Read the model definition and answer for the solid it produces. Units are mm, in the model's axes. Face numbers are marked on the shaded views. Coordinates: 2 decimals unless noted, no trailing zeros. Order: outer loops, then holes, each group sorted by start corner. A loop starts at its lowest first (then second) coordinate and runs counter-clockwise, first axis right, second up.
from build123d import *

# Parameters (mm, degrees)
SKETCH_1_W           = 52
SKETCH_1_H           = 95
EXTRUDE_1_DEPTH      = 180
SKETCH_2_W           = 23
SKETCH_2_H           = 90
CUT_EXTRUDE_1_DEPTH  = 140
SKETCH_3_W           = 9.5
SKETCH_3_H           = 2.2
CUT_EXTRUDE_2_DEPTH  = 140
CHAMFER_1_SIZE       = 2
CUT_EXTRUDE_3_DEPTH  = 140
SKETCH_5_W           = 140
SKETCH_5_H           = 15
CUT_EXTRUDE_4_DEPTH  = 140
SKETCH_6_W           = 140
SKETCH_6_H           = 15
CUT_EXTRUDE_7_DEPTH  = 140
CUT_EXTRUDE_8_DEPTH  = 140
SKETCH_8_W           = 24.808453611
SKETCH_8_H           = 15
CUT_EXTRUDE_9_DEPTH  = 140
SKETCH_9_W           = 10
SKETCH_9_H           = 14.176065277
SKETCH_9_H_2         = 15.630765607
CUT_EXTRUDE_10_DEPTH = 140
SKETCH_10_W          = 52
SKETCH_10_H          = 0.823934723
CUT_EXTRUDE_11_DEPTH = 10
SKETCH_12_R          = 3.01
EXTRUDE_2_DEPTH      = 20
CHAMFER_3_SIZE       = 0.5
SKETCH_13_R          = 3.01
EXTRUDE_4_DEPTH      = 20
CHAMFER_4_SIZE       = 0.5
EXTRUDE_START        = 20
SKETCH_15_R          = 3.01
EXTRUDE_5_DEPTH      = 20
CHAMFER_5_SIZE       = 0.5


with BuildPart() as part:
    # 草图1 → 凸台-拉伸1 (new body)
    with BuildSketch(Plane.XY):
        with Locations((0, 47.5)):
            Rectangle(SKETCH_1_W, SKETCH_1_H)
    extrude(amount=EXTRUDE_1_DEPTH)

    # 草图2 → 切除-拉伸1 (cut)
    with BuildSketch(Plane(origin=(0, 0, 0), x_dir=(-1, 0, 0), z_dir=(0, 0, -1))):
        with Locations((0, 50)):
            Rectangle(SKETCH_2_W, SKETCH_2_H)
    extrude(amount=-CUT_EXTRUDE_1_DEPTH, mode=Mode.SUBTRACT)

    # 草图3 → 切除-拉伸2 (cut)
    with BuildSketch(Plane(origin=(0, 0, 0), x_dir=(-1, 0, 0), z_dir=(0, 0, -1))):
        with Locations((-16.25, 6.1)):
            Rectangle(SKETCH_3_W, SKETCH_3_H)
        with Locations((16.25, 6.1)):
            Rectangle(SKETCH_3_W, SKETCH_3_H)
    extrude(amount=-CUT_EXTRUDE_2_DEPTH, mode=Mode.SUBTRACT)

    # 倒角1
    chamfer_1_edges = [part.edges().sort_by_distance(p)[0] for p in [
        (11.5, 51.1, 140),
        (0, 95, 140),
        (11.5, 95, 70),
        (-11.5, 95, 70),
        (11.5, 51.1, 0),
        (-11.5, 51.1, 140),
        (-11.5, 51.1, 0),
        (11.5, 7.2, 70),
        (16.25, 7.2, 140),
        (-16.25, 7.2, 140),
        (-11.5, 7.2, 70),
    ]]
    chamfer(chamfer_1_edges, length=CHAMFER_1_SIZE)

    # 草图4 → 切除-拉伸3 (cut)
    with BuildSketch(Plane(origin=(0, 0, 0), x_dir=(-1, 0, 0), z_dir=(0, 0, -1))):
        Polygon((-0.565514489, 0), (0, 0), (12.126296858, 0), (12.126296858, 5), (-11.873703142, 5), (-11.873703142, 0), align=None)
    extrude(amount=-CUT_EXTRUDE_3_DEPTH, mode=Mode.SUBTRACT)

    # 草图5 → 切除-拉伸4 (cut)
    with BuildSketch(Plane(origin=(26, 0, 0), x_dir=(0, 0, -1), z_dir=(1, 0, 0))):
        with Locations((-70, 87.5)):
            Rectangle(SKETCH_5_W, SKETCH_5_H)
    extrude(amount=-CUT_EXTRUDE_4_DEPTH, mode=Mode.SUBTRACT)

    # 草图6 → 切除-拉伸7 (cut)
    with BuildSketch(Plane(origin=(26, 0, 0), x_dir=(0, 0, -1), z_dir=(1, 0, 0))):
        with Locations((-70, 16.784197303)):
            Rectangle(SKETCH_6_W, SKETCH_6_H)
    extrude(amount=-CUT_EXTRUDE_7_DEPTH, mode=Mode.SUBTRACT)

    # 草图7 → 切除-拉伸8 (cut)
    with BuildSketch(Plane(origin=(0, 95, 0), x_dir=(1, 0, 0), z_dir=(0, 1, 0))):
        Polygon((0, -140), (21.6540992, -140), (21.6540992, -164.808453611), (-20.3459008, -164.808453611), (-20.926391083, -164.808453611), (-20.926391083, -140), align=None)
    extrude(amount=-CUT_EXTRUDE_8_DEPTH, mode=Mode.SUBTRACT)

    # 草图8 → 切除-拉伸9 (cut)
    with BuildSketch(Plane(origin=(26, 0, 0), x_dir=(0, 0, -1), z_dir=(1, 0, 0))):
        with Locations((-152.404226806, 87.5)):
            Rectangle(SKETCH_8_W, SKETCH_8_H)
        with Locations((-152.404226806, 16.784197303)):
            Rectangle(SKETCH_8_W, SKETCH_8_H)
    extrude(amount=-CUT_EXTRUDE_9_DEPTH, mode=Mode.SUBTRACT)

    # 草图9 → 切除-拉伸10 (cut)
    with BuildSketch(Plane(origin=(26, 0, 0), x_dir=(0, 0, -1), z_dir=(1, 0, 0))):
        with Locations((-169.808453611, 87.911967362)):
            Rectangle(SKETCH_9_W, SKETCH_9_H)
        with Locations((-169.808453611, 17.099580106)):
            Rectangle(SKETCH_9_W, SKETCH_9_H_2)
    extrude(amount=-CUT_EXTRUDE_10_DEPTH, mode=Mode.SUBTRACT)

    # 草图10 → 切除-拉伸11 (cut)
    with BuildSketch(Plane(origin=(0, 0, 164.808453611), x_dir=(-1, 0, 0), z_dir=(0, 0, -1))):
        with Locations((0, 80.411967362)):
            Rectangle(SKETCH_10_W, SKETCH_10_H)
    extrude(amount=-CUT_EXTRUDE_11_DEPTH, mode=Mode.SUBTRACT)

    # 草图12 → 凸台-拉伸2 (add)
    with BuildSketch(Plane.XY.offset(180)):
        with Locations(Location((0, 3.01, 0), (0, 0, 270))):
            Circle(SKETCH_12_R)
    extrude(amount=EXTRUDE_2_DEPTH)

    # 倒角3
    chamfer_3_edges = [part.edges().sort_by_distance(p)[0] for p in [
        (0, 6.02, 200),
    ]]
    chamfer(chamfer_3_edges, length=CHAMFER_3_SIZE)

    # 草图13 → 凸台-拉伸4 (add)
    with BuildSketch(Plane(origin=(26, 0, 0), x_dir=(0, 0, -1), z_dir=(1, 0, 0))):
        with Locations(Location((-25, 3.01, 0), (0, 0, 270))):
            Circle(SKETCH_13_R)
    extrude(amount=EXTRUDE_4_DEPTH)

    # 倒角4
    # the kernel refuses this chamfer: 0.5 mm, written as the material it adds along each edge
    with BuildSketch(Plane(origin=(26, 3.01, 25), x_dir=(0, -1, 0), z_dir=(0, 0, 1))) as chamfer_4_piece_1_section:
        Polygon((3.01 + CHAMFER_4_SIZE, 0), (3.01, CHAMFER_4_SIZE), (3.01, 0), align=None)
    chamfer_4_piece_1 = revolve(axis=Axis((26, 3.01, 25), (1, 0, 0)), mode=Mode.PRIVATE)
    chamfer_4_piece_1 = split(chamfer_4_piece_1, bisect_by=Plane(origin=(26.240420809, 0, 25), z_dir=(0, 1, 0)), keep=Keep.TOP, mode=Mode.PRIVATE)
    add(chamfer_4_piece_1)
    # the kernel refuses this chamfer: 0.5 mm, written as the material it takes off along each edge
    with BuildSketch(Plane(origin=(46, 3.01, 25), x_dir=(0, -1, 0), z_dir=(0, 0, 1))) as chamfer_4_2_piece_1:
        Polygon((3.01, -CHAMFER_4_SIZE), (3.01 - CHAMFER_4_SIZE, 0), (3.01, 0), align=None)
    revolve(axis=Axis((46, 3.01, 25), (1, 0, 0)), mode=Mode.SUBTRACT)

    # 草图15 → 凸台-拉伸5 (add)
    with BuildSketch(Plane.ZY.offset(26).offset(EXTRUDE_START)):
        with Locations(Location((25, 3.01, 0), (0, 0, 270))):
            Circle(SKETCH_15_R)
    extrude(amount=-EXTRUDE_5_DEPTH)

    # 倒角5
    # the kernel refuses this chamfer: 0.5 mm, written as the material it adds along each edge
    with BuildSketch(Plane(origin=(-26, 3.01, 25), x_dir=(0, -1, 0), z_dir=(0, 0, -1))) as chamfer_5_piece_1_section:
        Polygon((3.01 + CHAMFER_5_SIZE, 0), (3.01, CHAMFER_5_SIZE), (3.01, 0), align=None)
    chamfer_5_piece_1 = revolve(axis=Axis((-26, 3.01, 25), (-1, 0, 0)), mode=Mode.PRIVATE)
    chamfer_5_piece_1 = split(chamfer_5_piece_1, bisect_by=Plane(origin=(-26.240420809, 0, 25), z_dir=(0, 1, 0)), keep=Keep.TOP, mode=Mode.PRIVATE)
    add(chamfer_5_piece_1)
    # the kernel refuses this chamfer: 0.5 mm, written as the material it takes off along each edge
    with BuildSketch(Plane(origin=(-46, 3.01, 25), x_dir=(0, -1, 0), z_dir=(0, 0, -1))) as chamfer_5_2_piece_1:
        Polygon((3.01, -CHAMFER_5_SIZE), (3.01 - CHAMFER_5_SIZE, 0), (3.01, 0), align=None)
    revolve(axis=Axis((-46, 3.01, 25), (-1, 0, 0)), mode=Mode.SUBTRACT)


solid = part.part
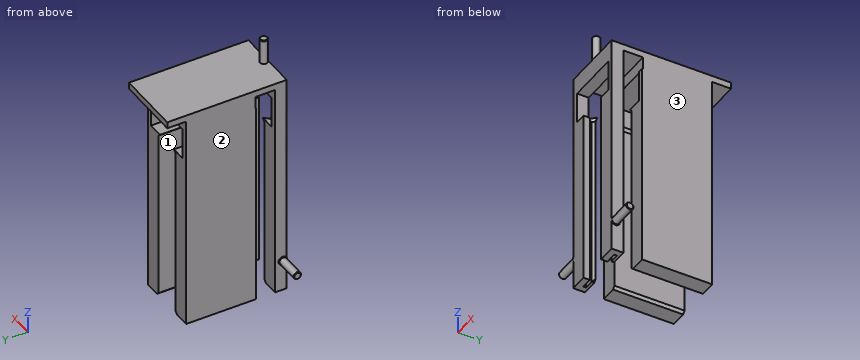
Q1. Straight lines are drawn through the part: L1, parallel to Y at x = 19, z = 107; L2, parallel to Y at x = -24, z = 16.5; L3, parallel to X at y = 78, z = 122.5. For each, find the intervals that lie inside material, in ascending order.
Q2. The part is cut by section A-A, the plane z = 85.5. Determine the outline of the cut face in (x, y).
Q3. Each of these flat-tipped pins is pushed along its axis until it touches: P1, Ø1.5, axis at y = 71, z = 78, coming from the -X side; P2, Ø9, axis at x = -15, y = 45.5, coming from the +Z side; P3, Ø4.5, axis at x = 3, y = 89.5, coming from the -Z side; P4, Ø12, axis at x = -1.5, z = 30, coming from the -Y side. Where does it stop, or does it pass through?
Q4. Determine the mould class of the marked faces 1, 2 and 3 for opening direction X: +X half, -X half, draft (parallel to the pull), parting line (faces both ways), or undercut.
Q5. The part is cut by section B-B, the plane x = -18. Determine the outline of the cut face in (y, z), then the cut area to 3 significant figures.
Q6. The part is cut by section C-C, the plane y = 70. Determine the outline of the cut face in (x, z).
Computed values:
1. L1: y = 0 to 5, 7.2 to 9.28, 24.28 to 80
1. L2: y = 0 to 9.28, 24.28 to 80
1. L3: x = -26 to -11.5, 11.5 to 26
2. outline: (-26, 0) - (-12.13, 0) - (-12.13, 5) - (-21, 5) - (-21, 7.2) - (-13.5, 7.2) - (-11.5, 9.2) - (-11.5, 9.28) - (-26, 9.28) - close; (-26, 24.28) - (-11.5, 24.28) - (-11.5, 80) - (-26, 80) - close; (11.5, 9.2) - (13.5, 7.2) - (21, 7.2) - (21, 5) - (11.87, 5) - (11.87, 0) - (26, 0) - (26, 9.28) - (11.5, 9.28) - close; (11.5, 24.28) - (26, 24.28) - (26, 80) - (11.5, 80) - close
3. P1: stops at x = -26
3. P2: stops at z = 180
3. P3: stops at z = 174.81
3. P4: passes through
4. face 1: undercut
4. face 2: -X half
4. face 3: +X half
5. outline: (0, 0) - (5, 0) - (5, 140) - (0, 140) - close; (0, 164.81) - (9.28, 164.81) - (9.28, 174.81) - (24.91, 174.81) - (24.91, 164.81) - (80, 164.81) - (80, 174.81) - (95, 174.81) - (95, 180) - (0, 180) - close; (5.2, 140) - (7.2, 138) - (7.2, 0) - (9.28, 0) - (9.28, 140) - close; (24.28, 0) - (80, 0) - (80, 140) - (24.28, 140) - close
5. area: 9,930 mm2
6. outline: (-26, 0) - (-13.5, 0) - (-11.5, 2) - (-11.5, 138) - (-9.5, 140) - (-20.93, 140) - (-20.93, 164.81) - (21.65, 164.81) - (21.65, 140) - (9.5, 140) - (11.5, 138) - (11.5, 2) - (13.5, 0) - (26, 0) - (26, 180) - (-26, 180) - close
